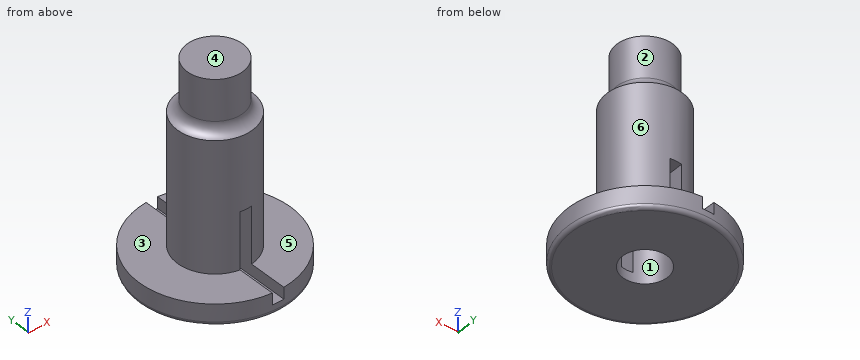
from build123d import *

# Parameters (mm, degrees)
SKETCH1_R               = 197.5
BOSS_EXTRUDE1_DEPTH     = 55
SKETCH2_R               = 97.5
BOSS_EXTRUDE2_DEPTH     = 335
SKETCH3_R               = 72.5
BOSS_EXTRUDE3_DEPTH     = 470
CUT_EXTRUDE1_DEPTH      = 30
CUT_EXTRUDE2_DEPTH      = 15
CUT_EXTRUDE2_DEPTH_BACK = 15
CUT_EXTRUDE3_DEPTH      = 235
CUT_EXTRUDE3_DEPTH_BACK = 285
SKETCH8_R               = 57.5
FILLET1_R               = 30
FILLET2_R               = 10


with BuildPart() as part:
    # Sketch1 → Boss-Extrude1 (new body)
    with BuildSketch(Plane.XY):
        Circle(SKETCH1_R)
    extrude(amount=-BOSS_EXTRUDE1_DEPTH)

    # Sketch2 → Boss-Extrude2 (add)
    with BuildSketch(Plane.XY):
        Circle(SKETCH2_R)
    extrude(amount=BOSS_EXTRUDE2_DEPTH)

    # Sketch3 → Boss-Extrude3 (add)
    with BuildSketch(Plane.XY):
        with Locations(Location((0, 0, 0), (0, 0, 180))):
            Circle(SKETCH3_R)
    extrude(amount=BOSS_EXTRUDE3_DEPTH)

    # Sketch4 → Cut-Extrude1 (cut)
    with BuildSketch(Plane.XY):
        Polygon((0, 197.5), (-15, 197.5), (-15, -197.5), (0, -197.5), (15, -197.5), (15, 197.5), align=None)
    extrude(amount=-CUT_EXTRUDE1_DEPTH, mode=Mode.SUBTRACT)

    # Sketch7 → Cut-Extrude2 (cut, two sides: drawn at the far end of the back side and taken through both)
    with BuildSketch(Plane(origin=(0, 0, 0), x_dir=(0, 0, -1), z_dir=(1, 0, 0)).offset(-CUT_EXTRUDE2_DEPTH_BACK)):
        Polygon((0, 0), (0, 273), (-161.375, 273), (-138.625, -273), (0, -273), align=None)
    extrude(amount=CUT_EXTRUDE2_DEPTH + CUT_EXTRUDE2_DEPTH_BACK, mode=Mode.SUBTRACT)

    # Sketch8 → Cut-Extrude3 (cut, two sides: drawn at the far end of the back side and taken through both)
    with BuildSketch(Plane.XY.offset(-CUT_EXTRUDE3_DEPTH_BACK)):
        Circle(SKETCH8_R)
    extrude(amount=CUT_EXTRUDE3_DEPTH + CUT_EXTRUDE3_DEPTH_BACK, mode=Mode.SUBTRACT)

    # Fillet1
    # the kernel refuses this fillet: 30 mm, written as the material it adds along each edge
    with BuildSketch(Plane(origin=(0, 0, 335), x_dir=(-1, 0, 0), z_dir=(0, -1, 0))) as fillet1_piece_1:
        with BuildLine():
            CenterArc((102.5, -29.580398916), FILLET1_R, 99.594068227, 80.405931773)
            Line((72.5, -29.580398916), (71.9, -29.580398916))
            Line((71.9, -29.580398916), (71.9, 0))
            Line((71.9, 0), (72.5, 0.6))
            ThreePointArc((72.5, 0.6), (85, 0.6), (97.4, 0.591607978))
            Line((97.4, 0.591607978), (97.5, 0))
        make_face()
    revolve(axis=Axis((0, 0, 335), (0, 0, -1)))

    # Fillet2
    fillet2_edges = [part.edges().sort_by_distance(p)[0] for p in [
        (-197.5, 0, -55),
    ]]
    fillet(fillet2_edges, radius=FILLET2_R)


solid = part.part
Verification items for the finished model (mm, model axes). Face numbers are marked on the shaded views. A direction names the side the tool comes from. Give positions to 0.01 mm unless a question says otherwise; leave off trailing zeros. Write each loop counter-clockwise with the first axis right and the second up, starting at its lowest first coordinate (ties: lowest second). Pieces come first, ordered by that corner, then holes. Notation, with made-up numbers: (65, -38.5) - (71, -38.5) arc R10 cw to (71, -34.5) - close; hole circle Ø4 at (35.25, 6). An arc over 180 degrees is marked (long way). Answer as CSV lines item,"result". Start each with the question number.
1. Depth check by flat-ended pin: pin 1 (9 mm diameter, centred on x = 6, y = 126.5, fed in from +Z); pin 2 (2 mm diameter, centred on y = 24, z = 83.5, fed in from -X); pin 3 (6 mm diameter, centred on x = -20, y = 20, fed in from -Z). Enter the tip coordinate at first touch or a pass-through.
2. Sectioned sample at B-B (x = 0). Record the boundary of the cut face in (y, z).
3. Sectioned sample at C-C (y = 0). Record the boundary of the cut face in (x, z).
4. Sectioned sample at D-D (z = 193.5). Record the boundary of the cut face in (x, y), then the cut area to 3 significant figures.
5. Set-up check for the marked faces 4, 5 and 6: record each of +Z, -Z, +X, -X, +Y, -Y from which the full face is reachable in a straight line by a thin tool's end or side.
6. Draft check along Y on the marked faces 1, 2 and 3. Enter one of: pulls with the +Y half, pulls with the -Y half, needs draft (parallel to the pull), parting line crosses it, or undercut.
7. Sectioned sample at A-A (z = 86). Record the boundary of the cut face in (x, y).
8. Thickness scan on line 1 (Y direction, x = 0, z = 160); line 2 (Z direction, x = -14, y = -125.5). Record the ranges inside material, lowest first.
Derived:
1,pin 1,"z = -30"
1,pin 2,"x = -94.75"
1,pin 3,"z = 235"
2,outline,"(-197.5, -45) arc R10 ccw to (-187.5, -55) - (-57.5, -55) - (-57.5, -30) - (-197.5, -30) - close; (-97.5, 145.94) - (-57.5, 147.6) - (-57.5, 235) - (57.5, 235) - (57.5, 152.4) - (97.5, 154.06) - (97.5, 335) arc R30 cw to (72.5, 364.58) - (72.5, 470) - (-72.5, 470) - (-72.5, 364.58) arc R30 cw to (-97.5, 335) - close; (57.5, -55) - (187.5, -55) arc R10 ccw to (197.5, -45) - (197.5, -30) - (57.5, -30) - close"
3,outline,"(-197.5, -45) arc R10 ccw to (-187.5, -55) - (-57.5, -55) - (-57.5, 235) - (57.5, 235) - (57.5, -55) - (187.5, -55) arc R10 ccw to (197.5, -45) - (197.5, 0) - (97.5, 0) - (97.5, 335) arc R30 cw to (72.5, 364.58) - (72.5, 470) - (-72.5, 470) - (-72.5, 364.58) arc R30 cw to (-97.5, 335) - (-97.5, 0) - (-197.5, 0) - close"
4,outline,"circle Ø195 at (0, 0); hole circle Ø115 at (0, 0)"
4,area,"19,500 mm²"
5,face 4,"+Z, +X, -X, +Y, -Y"
5,face 5,"+Z, +X"
5,face 6,"+Z"
6,face 1,"undercut"
6,face 2,"parting line crosses it"
6,face 3,"needs draft"
7,outline,"(-15, -96.34) - (-15, -55.51) arc R57.5 cw to (-15, 55.51) - (-15, 96.34) arc R97.5 ccw to start; (15, -96.34) arc R97.5 ccw to (15, 96.34) - (15, 55.51) arc R57.5 cw to (15, -55.51) - close"
8,line 1,"-97.5 to -57.5, 57.5 to 97.5"
8,line 2,"-55 to -30"
